Study the drawing (mm; zero at the part's minimum x, y, z) and answer. A direction names the side the tool comes from. Coordinates: 2 decimals unless noted, no trailing zeros. Order: outer loops, then holes, each group sorted by start corner. A loop starts at its lowest first (then second) coordinate and runs counter-clockwise, first axis right, second up. Notation, with made-up numbers: (-9, 10) -> (46, 10) arc R26 ccw to (46, 45) -> close; hole circle Ø10 at (37.25, -26). An arc over 180 degrees is marked (long way). One line per question, with ' | ' between items.
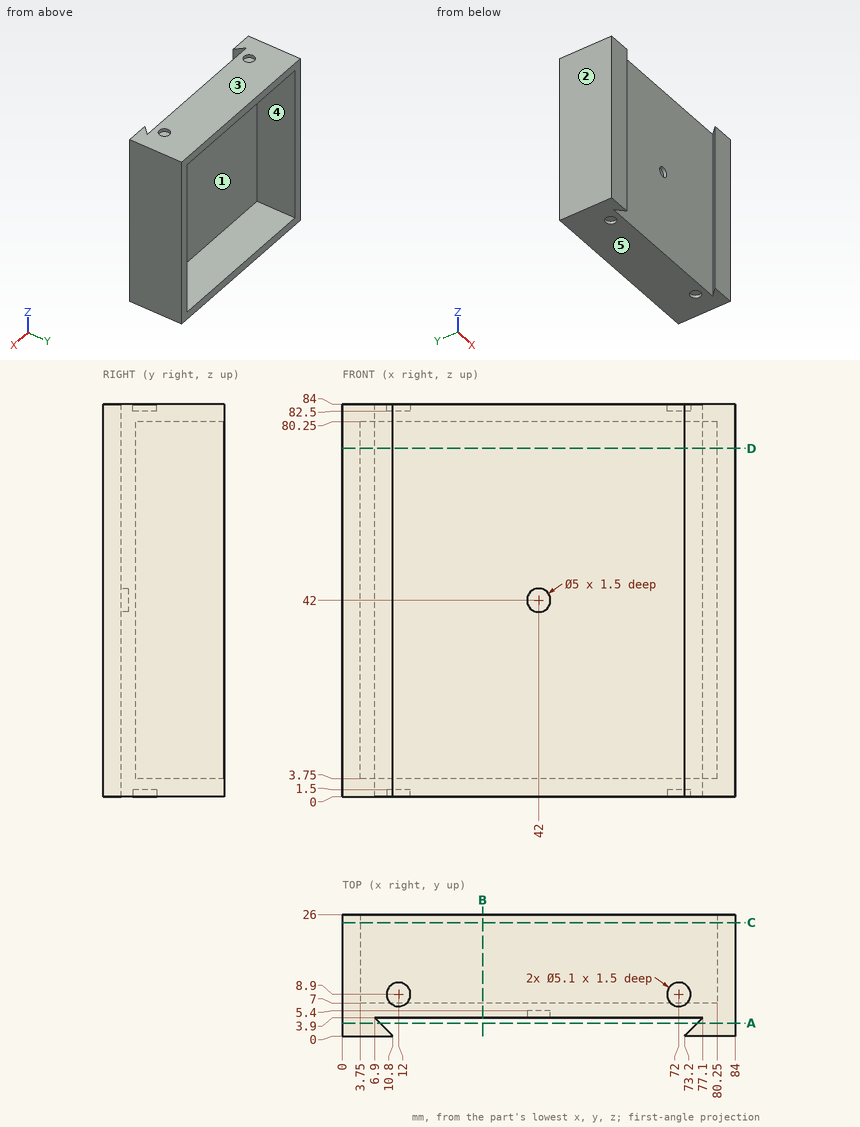
Item 1: Section A-A, the plane y = 2.75 is taken. Give the vertices of the cut face in (x, z).
Computed values:
outline: (0, 0) -> (8.05, 0) -> (8.05, 84) -> (0, 84) -> close; (75.95, 0) -> (84, 0) -> (84, 84) -> (75.95, 84) -> close
Item 2: For the marked faces 4 and 5, determine the directions among +Z, -Z, +X, -X, +Y, -Y from which every point of the face is accessible in a straight line to the end or side of a thin tool.
Computed values:
face 4: +Y | face 5: -Z, +X, -X, +Y, -Y
Item 3: Each of these flat-tipped pins is pushed along its axis until it touches: pin 1 Ø5.5 at (x, y) = (11.5, 8) entering from +Z; pin 2 Ø2 at (x, z) = (46.5, 73.5) entering from -Y; pin 3 Ø2.5 at (x, y) = (72.5, 8) entering from -Z; pin 4 Ø6 at (x, z) = (74.5, 53.5) entering from +Y. Where does it stop, or does it pass through?
Computed values:
pin 1: stops at z = 84 | pin 2: stops at y = 3.9 | pin 3: stops at z = 1.5 | pin 4: stops at y = 7
Item 4: Section B-B, the plane x = 30 is taken. Give the vertices of the cut face in (y, z).
Computed values:
outline: (3.9, 0) -> (26, 0) -> (26, 3.75) -> (7, 3.75) -> (7, 80.25) -> (26, 80.25) -> (26, 84) -> (3.9, 84) -> close
Item 5: Section C-C, the plane y = 24.25 is taken. Give the vertices of the cut face in (x, z).
Computed values:
outline: (0, 0) -> (84, 0) -> (84, 84) -> (0, 84) -> close; hole (3.75, 3.75) -> (80.25, 3.75) -> (80.25, 80.25) -> (3.75, 80.25) -> close
Item 6: Determine the mould class of the marked faces 1, 2 and 3 for opening direction Z: pulls with the +Z half, pulls with the -Z half, needs draft (parallel to the pull), parting line crosses it, or undercut.
Computed values:
face 1: undercut | face 2: needs draft | face 3: pulls with the +Z half
Item 7: Find the intervals of material crossed by L1, parallel to Z at x = 42, y = 4.7; L2, parallel to Y at x = 12, z = 1.15; L3, parallel to X at y = 8.5, z = 30, in increasing order.
Computed values:
L1: z = 0 to 39.5, 44.5 to 84 | L2: y = 3.9 to 6.35, 11.45 to 26 | L3: x = 0 to 3.75, 80.25 to 84
Item 8: Section D-D, the plane z = 74.5 is taken. Give the vertices of the cut face in (x, y).
Computed values:
outline: (0, 0) -> (10.8, 0) -> (6.9, 3.9) -> (77.1, 3.9) -> (73.2, 0) -> (84, 0) -> (84, 26) -> (80.25, 26) -> (80.25, 7) -> (3.75, 7) -> (3.75, 26) -> (0, 26) -> close
